Check sheet for the modelled part. Datum: model origin and axes. Units: mm. Give positions to 0.01 mm unless a question says otherwise; leave off trailing zeros. Order: outer loops, then holes, each group sorted by start corner. A loop starts at its lowest first (then second) coordinate and runs counter-clockwise, first axis right, second up.
from build123d import *

# Parameters (mm, degrees)
F1_DEPTH = 43.434
F3_DEPTH = 43.435


with BuildPart() as f1:
    # F0 (on Top) → F1 (new body)
    with BuildSketch(Plane.XY):
        Polygon((0, 37.737992), (-52.417379, 37.737992), (-52.417379, 0), (52.417379, 0), (52.417379, 37.737992), align=None)
    extrude(amount=F1_DEPTH)

    # F2 (on face) → F3 (cut, through all)
    with BuildSketch(Plane.XY.offset(43.434)):
        with BuildLine():
            Line((-33.308111, 0), (33.308111, 0))
            ThreePointArc((33.308111, 0), (0, 33.308111), (-33.308111, 0))
        make_face()
    extrude(amount=-F3_DEPTH, mode=Mode.SUBTRACT)


solid = f1.part
1) Section check C-C, the plane x = 0. Record the cut outline in (y, z).
Recorded:
outline: (33.31, 0) - (37.74, 0) - (37.74, 43.43) - (33.31, 43.43) - close
2) Section check B-B, the plane z = 3. Record the cut outline in (x, y), then the cut area to 3 significant figures.
Recorded:
outline: (-52.42, 0) - (-33.31, 0) arc R33.31 cw to (33.31, 0) - (52.42, 0) - (52.42, 37.74) - (-52.42, 37.74) - close
area: 2,210 mm2
3) Section check D-D, the plane y = 8. Record the cut outline in (x, z), then the cut area to 3 significant figures.
Recorded:
outline: (-52.42, 0) - (-32.33, 0) - (-32.33, 43.43) - (-52.42, 43.43) - close; (32.33, 0) - (52.42, 0) - (52.42, 43.43) - (32.33, 43.43) - close
area: 1,740 mm2
4) Section check A-A, the plane y = 12.5. Record the cut outline in (x, z), then the cut area to 3 significant figures.
Recorded:
outline: (-52.42, 0) - (-30.87, 0) - (-30.87, 43.43) - (-52.42, 43.43) - close; (30.87, 0) - (52.42, 0) - (52.42, 43.43) - (30.87, 43.43) - close
area: 1,870 mm2
5) Material ranges on L1, parallel to X at y = 20, z = 25; L2, parallel to X at y = 27.5, z = 14.5; L3, parallel to Y at x = -20, z = 30.5, recorded low to high.
Recorded:
L1: x = -52.42 to -26.64, 26.64 to 52.42
L2: x = -52.42 to -18.79, 18.79 to 52.42
L3: y = 26.64 to 37.74
6) Draft check along X on faces 1 (the face through (-52.417, 19, 21)), 2 (the face through (0.7, 33.3, 22)), 3 (the face through (52.417, 19, 21)), 4 (the face through (1, 37.738, 21)). Enter one of: +X half, -X half, draft (parallel to the pull), parting line (faces both ways), or undercut.
Recorded:
face 1: -X half
face 2: undercut
face 3: +X half
face 4: draft
7) Depth check by flat-ended pin: pin 1 Ø10 at (x, y) = (-12.5, 22) entering from -Z. Enter the tip coordinate at first touch or a pass-through.
Recorded:
pin 1: passes through
